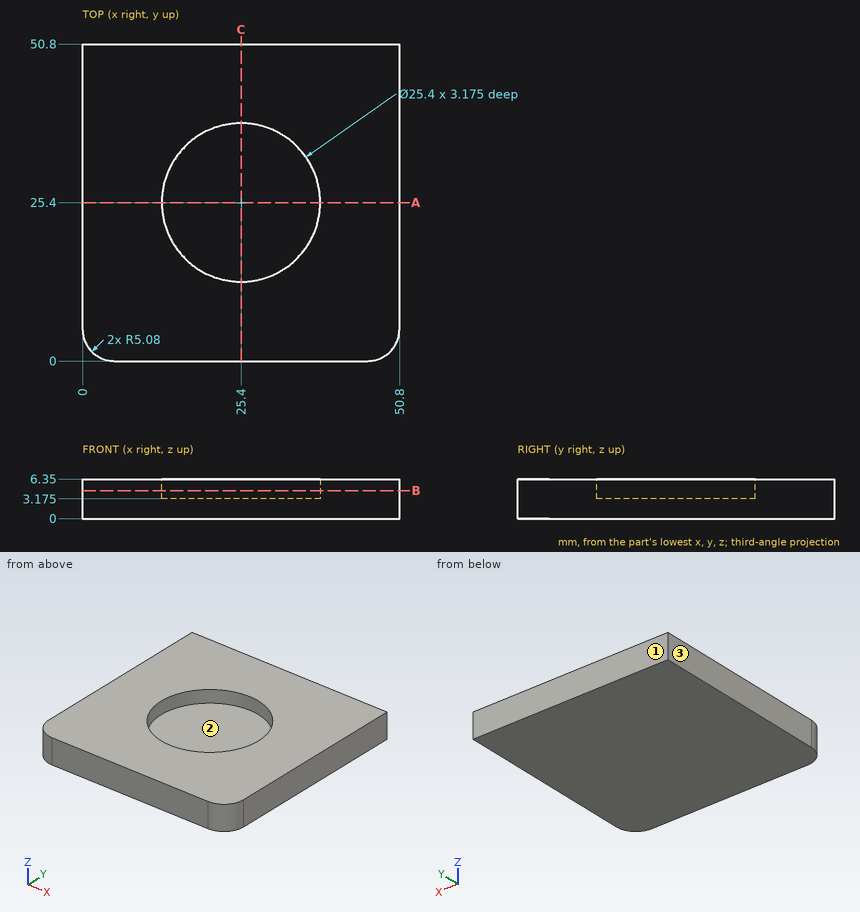
Print and shaded views of the part. All mm, measured from the part's lowest x, y and z. Give positions to 0.01 mm unless a question says otherwise; leave off trailing zeros. Order: outer loops, then holes, each group sorted by start corner. A loop starts at its lowest first (then second) coordinate and runs counter-clockwise, first axis right, second up. Notation, with made-up numbers: (-8.5, 4) - (8.5, 4) arc R3 cw to (8.5, 8) - close; hole circle Ø8 at (25, 65). An arc over 180 degrees is marked (long way). One line per item, written item: value.
Item 1: Pin check, flat tip, straight feed: pin 1 Ø20.5 at (x, y) = (25.4, 25.4) entering from +Z (3 decimals). Stop position of the tip, or through.
Response values:
pin 1: z = 3.175
Item 2: Slice it at B-B (z = 4.5). List the corners of the cut face in (x, y).
Response values:
outline: (0, 5.08) arc R5.08 ccw to (5.08, 0) - (45.72, 0) arc R5.08 ccw to (50.8, 5.08) - (50.8, 50.8) - (0, 50.8) - close; hole circle Ø25.4 at (25.4, 25.4)
Item 3: Slice it at A-A (y = 25.4). List the corners of the cut face in (x, z) (3 decimals), then the cut area to 3 significant figures.
Response values:
outline: (0, 0) - (50.8, 0) - (50.8, 6.35) - (38.1, 6.35) - (38.1, 3.175) - (12.7, 3.175) - (12.7, 6.35) - (0, 6.35) - close
area: 242 mm2
Item 4: Two-plate mould, pull along X, no slides. Class the marked faces 1, 2 and 3: released by +X, released by -X, zero draft, split by the parting line, or undercut.
Response values:
face 1: zero draft
face 2: undercut
face 3: released by -X
Item 5: Wall check: line 1 (Y direction, x = 25.4, z = 5.6); line 2 (Z direction, x = 33, y = 28) (3 decimals); line 3 (Y direction, x = 5, z = 5.5). Give the ranges that are in metal, low to high.
Response values:
line 1: 0 to 12.7, 38.1 to 50.8
line 2: 0 to 3.175
line 3: 0 to 50.8
